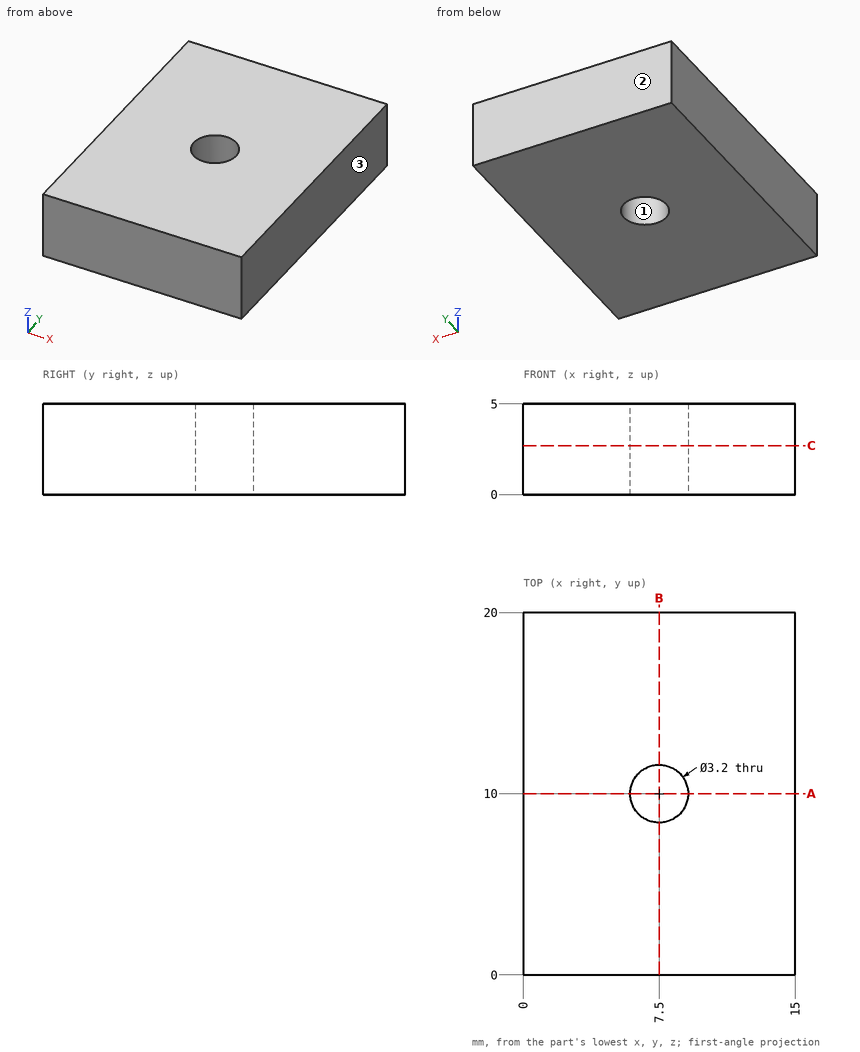
The drawing under review shows one solid part. Ordinate dimensions are in mm from its lowest x, y, z. Coordinates: 2 decimals unless noted, no trailing zeros. Order: outer loops, then holes, each group sorted by start corner. A loop starts at its lowest first (then second) coordinate and runs counter-clockwise, first axis right, second up. Notation, with made-up numbers: (-34.5, -38) - (14.5, -38) arc R13 cw to (14.5, -26) - close; hole circle Ø11 at (85, -15.5). An arc over 180 degrees is marked (long way). Put each result on its own line as item: value.
1) Take a section at A-A, the plane y = 10. Give the boundary of the cut face in (x, z).
Response values:
outline: (0, 0) - (5.9, 0) - (5.9, 5) - (0, 5) - close; (9.1, 0) - (15, 0) - (15, 5) - (9.1, 5) - close
2) The part is to be moulded in two halves that separate along X. For the marked faces 1, 2 and 3, say which applies: released by +X, released by -X, zero draft, split by the parting line, or undercut.
Response values:
face 1: undercut
face 2: zero draft
face 3: released by +X
3) Take a section at C-C, the plane z = 2.7. Give the boundary of the cut face in (x, y).
Response values:
outline: (0, 0) - (15, 0) - (15, 20) - (0, 20) - close; hole circle Ø3.2 at (7.5, 10)
4) Take a section at B-B, the plane x = 7.5. Give the boundary of the cut face in (y, z), and give its area (3 significant figures).
Response values:
outline: (0, 0) - (8.4, 0) - (8.4, 5) - (0, 5) - close; (11.6, 0) - (20, 0) - (20, 5) - (11.6, 5) - close
area: 84.0 mm²
5) Wall thickness on L1, parallel to Y at x = 7.5, z = 1.5; L2, parallel to Y at x = 8.5, z = 1.65: over which ranges is each line inside the solid? List them lowest first. Write a range as from..to.
Response values:
L1: y = 0..8.4, 11.6..20
L2: y = 0..8.75, 11.25..20
